CAD build for the part. Positions are in the model's coordinates, mm. Give positions to 0.01 mm unless a question says otherwise; leave off trailing zeros. Order: outer loops, then holes, each group sorted by start corner. A loop starts at its lowest first (then second) coordinate and runs counter-clockwise, first axis right, second up. Notation, with made-up numbers: (38.5, 62.25) -> (86.5, 62.25) arc R19 cw to (86.5, 74.25) -> close; hole circle Ø10 at (-25, -10). An arc over 180 degrees is marked (long way). Answer as CSV lines item,"result".
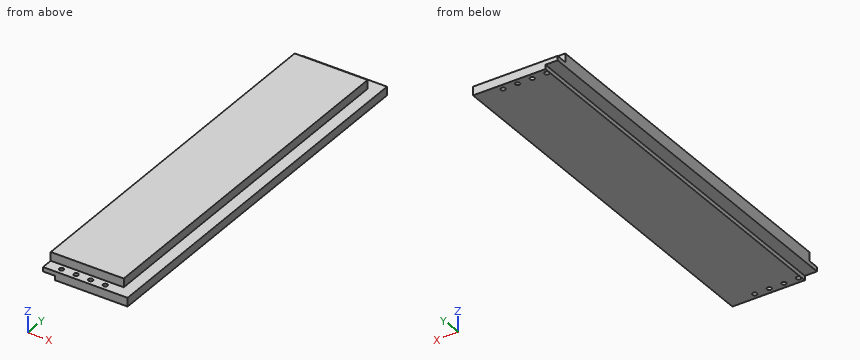
```python
from build123d import *

# Parameters (mm, degrees)
SKETCH1_W             = 92.7
SKETCH1_H             = 19.05
BOSS_EXTRUDE1_DEPTH   = 425.45
SKETCH2_W             = 9.525
SKETCH2_H             = 12.7
CUT_EXTRUDE1_DEPTH    = 436.716109536
SKETCH3_W             = 12.7
SKETCH3_H             = 9.525
CUT_EXTRUDE2_DEPTH    = 419.595052861
F_8_CLEARANCE_HOLE1_D = 4.9149
SKETCH6_W             = 13.335
SKETCH6_H             = 4.7498
CUT_EXTRUDE5_DEPTH    = 436.848477111


with BuildPart() as part:
    # Sketch1 → Boss-Extrude1 (new body)
    with BuildSketch(Plane(origin=(0, 0, 0), x_dir=(1, 0, 0), z_dir=(0, 1, 0))):
        with Locations((-21.55964711, -6.208264412)):
            Rectangle(SKETCH1_W, SKETCH1_H)
    extrude(amount=BOSS_EXTRUDE1_DEPTH)

    # Sketch2 → Cut-Extrude1 (cut, through all)
    with BuildSketch(Plane(origin=(24.79035289, 0, 0), x_dir=(0, 0, -1), z_dir=(1, 0, 0))):
        with Locations((-10.970764412, 419.1)):
            Rectangle(SKETCH2_W, SKETCH2_H)
        with Locations((-10.970764412, 6.35)):
            Rectangle(SKETCH2_W, SKETCH2_H)
    extrude(amount=-CUT_EXTRUDE1_DEPTH, mode=Mode.SUBTRACT)

    # Sketch3 → Cut-Extrude2 (cut, through all)
    with BuildSketch(Plane.XZ.offset(-12.7)):
        with Locations((18.44035289, 10.970764412)):
            Rectangle(SKETCH3_W, SKETCH3_H)
    extrude(amount=-CUT_EXTRUDE2_DEPTH, mode=Mode.SUBTRACT)

    # #8 Clearance Hole1 (through all)
    with Locations(Plane.XY.offset(6.208264412)):
        with Locations((-51.91764711, 6.35), (-35.91564711, 6.35), (-19.91364711, 6.35), (-3.91164711, 6.35), (-51.91764711, 419.1), (-35.91564711, 419.1), (-19.91364711, 419.1), (-3.91164711, 419.1)):
            Hole(F_8_CLEARANCE_HOLE1_D / 2)

    # Sketch6 → Cut-Extrude5 (cut, through all)
    with BuildSketch(Plane(origin=(-67.90964711, 425.45, -3.316735588), x_dir=(1, 0, 0), z_dir=(0, -1, 0))):
        with Locations((6.6675, 2.3749)):
            Rectangle(SKETCH6_W, SKETCH6_H)
    extrude(amount=CUT_EXTRUDE5_DEPTH, mode=Mode.SUBTRACT)


solid = part.part
```
1) Wall check: line 1 along X through (y, z) = (419.1, 3.5); line 2 along Y through (x, z) = (-27.5, 10.25); line 3 along X through (y, z) = (363.5, -1.5). Give the ranges that are in metal, low to high. Write a range as [from, to].
Data:
line 1,"x = [-67.91, -54.38], [-49.46, -38.37], [-33.46, -22.37], [-17.46, -6.37], [-1.45, 24.79]"
line 2,"y = [12.7, 412.75]"
line 3,"x = [-54.57, 24.79]"
2) Band-saw the part on B-B, the plane z = 12. Write the cut outline in (x, y), then the cut area to 3 significant figures.
Data:
outline,"(-67.91, 12.7) -> (12.09, 12.7) -> (12.09, 412.75) -> (-67.91, 412.75) -> close"
area,"32,000 mm2"
3) Band-saw the part on A-A, the plane y = 26. Write the cut outline in (x, z).
Data:
outline,"(-67.91, 1.43) -> (-54.57, 1.43) -> (-54.57, -3.32) -> (24.79, -3.32) -> (24.79, 6.21) -> (12.09, 6.21) -> (12.09, 15.73) -> (-67.91, 15.73) -> close"
4) Pin check, flat tips, straight feed: P1, Ø3, axis at x = 2, z = 10.5, coming from the +Y side; P2, Ø1.5, axis at y = 250.5, z = 13, coming from the +X side; P3, Ø5.5, axis at x = -51.92, y = 419.1, coming from the +Z side. Stop position of each tip, or through.
Data:
P1,"stops at y = 412.75"
P2,"stops at x = 12.09"
P3,"stops at z = 6.21"
